Autodesk Inventor part; units mm, degrees
ref_plane "YZ Plane" through (0, 0, 0) normal (1, 0, 0) x (0, 1, 0)
ref_plane "XZ Plane" through (0, 0, 0) normal (0, 1, 0) x (-1, 0, 0)
ref_plane "XY Plane" through (0, 0, 0) normal (0, 0, 1) x (1, 0, 0)
sketch "Sketch1" plane through (0, 0, 0) normal (0, 0, 1) x (1, 0, 0)
  circle A0 centre (0, 0) radius 101.6
  dimension "d10" = 203.2
extrude "Extrusion1" add sketch "Sketch1" along normal blind 90
sketch "Sketch2" plane through (0, 0, 90) normal (0, 0, 1) x (1, 0, 0)
  circle A0 centre (0, 63.5) radius 30.226
  circle A1 centre (-54.9926, -31.75) radius 30.226
  circle A2 centre (54.9926, -31.75) radius 30.226
  point P0 (0, 0)
  dimension "d4" = 360
  dimension "d11" = 63.5
  dimension "d12" = 60.452
extrude "Extrusion2" cut sketch "Sketch2" against normal blind 2
sketch "Sketch5" plane through (0, 0, 0) normal (0, 0, -1) x (-1, 0, 0)
  circle A0 centre (0, 0) radius 88.9
  dimension "d13" = 177.8
extrude "Extrusion4" add sketch "Sketch5" along normal blind 1.5
sketch "Sketch6" plane through (0, 0, 90) normal (0, 0, 1) x (1, 0, 0)
  circle A0 centre (54.9926, -31.75) radius 30.226
  circle A1 centre (54.9926, -31.75) radius 12.7
  circle A2 centre (0, 63.5) radius 12.7
  circle A3 centre (-54.9926, -31.75) radius 12.7
  point P0 (0, 0)
  dimension "d16" = 25.4
  dimension "d19" = 360
extrude "Extrusion5" cut sketch "Sketch6" against normal blind 53.8 contours A1 | A2 | A3
properties part number "membrane_mold"
Verification items for the finished model (mm, model axes). A direction names the side the tool comes from. Give positions to 0.01 mm unless a question says otherwise; leave off trailing zeros. Loops run counter-clockwise (first coordinate to the right, second up) from the corner with the lowest first, then second, coordinate; pieces in that order, holes last. Notation, with made-up numbers: (71.25, 6) - (119.25, 6) arc R19 ccw to (119.25, 22) - close; hole circle Ø4 at (47.5, 59.25). An arc over 180 degrees is marked (long way). Write each question's results on one line, items separated by ' | '.
1) Mould release check, pull along Y, two halves, no side actions. Record for faces 3 (the flat face through (0, -90, 0)), 4 (the cylindrical face through (-84.795, -26.703, -0.74)), 5 (the cylindrical face through (68.94, -58.566, 89.014)): pulls with the +Y half, pulls with the -Y half, needs draft (parallel to the pull), parting line crosses it, or undercut.
Solution:
face 3: needs draft | face 4: parting line crosses it | face 5: undercut
2) Material ranges on L1, parallel to X at y = 0.5, z = 81; L2, parallel to Z at x = -57, y = -29; L3, parallel to Y at x = -10.5, z = 57.5, recorded low to high. Write a range as from..to.
Solution:
L1: -101.6..101.6 | L2: -1.5..36.2 | L3: -101.06..56.36, 70.64..101.06
3) Sectioned sample at C-C on z = 82. Record the boundary of the cut face in (x, y).
Solution:
outline: circle Ø203.2 at (0, 0); hole circle Ø25.4 at (-54.99, -31.75); hole circle Ø25.4 at (0, 63.5); hole circle Ø25.4 at (54.99, -31.75)
4) Tool access check on faces 1 (the cylindrical face through (-1.653, 76.092, 62.463)), 2 (the cylindrical face through (-22.025, 99.184, 44.37)). Record the directions out of +Z, -Z, +X, -X, +Y, -Y that give a thin tool (end or side, any length) a straight path to the whole face; none if there is none.
Solution:
face 1: +Z | face 2: +Z, -Z
5) Sectioned sample at A-A on x = 0. Record the boundary of the cut face in (y, z), plus the area to 3 significant figures.
Solution:
outline: (-101.6, 0) - (-88.9, 0) - (-88.9, -1.5) - (88.9, -1.5) - (88.9, 0) - (101.6, 0) - (101.6, 90) - (93.73, 90) - (93.73, 88) - (76.2, 88) - (76.2, 36.2) - (50.8, 36.2) - (50.8, 88) - (33.27, 88) - (33.27, 90) - (-101.6, 90) - close | area: 17,100 mm2
6) Sectioned sample at D-D on x = 72. Record the boundary of the cut face in (y, z), plus the area to 3 significant figures.
Solution:
outline: (-71.68, 0) - (-52.15, 0) - (-52.15, -1.5) - (52.15, -1.5) - (52.15, 0) - (71.68, 0) - (71.68, 90) - (-6.76, 90) - (-6.76, 88) - (-56.74, 88) - (-56.74, 90) - (-71.68, 90) - close | area: 13,000 mm2
7) Sectioned sample at B-B on y = 63.5. Record the boundary of the cut face in (x, z).
Solution:
outline: (-79.31, 0) - (-62.22, 0) - (-62.22, -1.5) - (62.22, -1.5) - (62.22, 0) - (79.31, 0) - (79.31, 90) - (30.23, 90) - (30.23, 88) - (12.7, 88) - (12.7, 36.2) - (-12.7, 36.2) - (-12.7, 88) - (-30.23, 88) - (-30.23, 90) - (-79.31, 90) - close
8) Depth check by flat-ended pin: P1, Ø4, axis at x = -31, z = 18.5, coming from the -Y side; P2, Ø18, axis at x = 48.5, y = -43, coming from the +Z side; P3, Ø10, axis at y = 50, z = 15, coming from the -X side. Enter the tip coordinate at first touch or a pass-through.
Solution:
P1: y = -97.37 | P2: z = 88 | P3: x = -91.09
